Can you work these out from the model? Positions are in its coordinate system, mm. Face numbers are marked on the shaded views. Give positions to 0.01 mm unless a question says otherwise; leave off trailing zeros. Order: outer loops, then holes, each group sorted by start corner. A loop starts at its lowest first (then second) coordinate and runs counter-clockwise, first axis right, second up.
Item 1: I want a section at A-A, the plane x = 21.5. Write out the boundary of the cut face in (y, z).
Item 2: I'm going to push a flat-ended pin straight in: pin 1 Ø1.8 at (x, y) = (30, 6) entering from +Z. Where does the tip first touch, or does it pass through?
Item 3: If I drill on line 1 along X through (y, z) = (29, 1.4); line 2 along Y through (x, z) = (5, 3.65); line 3 along Y through (x, z) = (29, 0.5), over which ranges is the centre line in solid material (lowest first)?
Item 4: I want a section at D-D, the plane y = 5. Write out the boundary of the cut face in (x, z), then the cut area to 3 significant figures.
Item 5: If we mould it in two halves opening along Y, with no side actions, what happens to the marked faces 1, 2 and 3? For each: +Y half, -Y half, draft (parallel to the pull), parting line (faces both ways), or undercut.
Item 6: I want a section at B-B, the plane y = 17. Write out the boundary of the cut face in (x, z).
Item 7: I want a section at C-C, the plane z = 0.45. Write out the boundary of the cut face in (x, y), then the cut area to 3 significant figures.
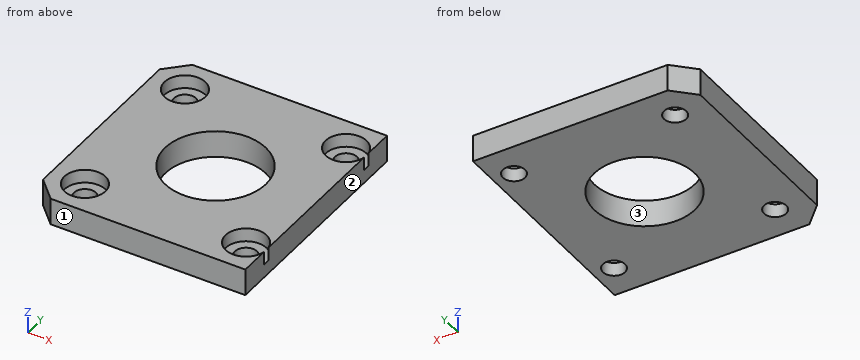
```python
from build123d import *

# Parameters (mm, degrees)
SKETCH_1_R          = 7.5
SKETCH_1_R_2        = 1.65
EXTRUDE_1_DEPTH     = 4
SKETCH_2_R          = 3.05
CUT_EXTRUDE_1_DEPTH = 2


with BuildPart() as part:
    # 草图1 → 凸台-拉伸1 (new body)
    with BuildSketch(Plane.XY):
        Polygon((0, 31), (3, 34), (32, 34), (32, 0), (3, 0), (0, 3), align=None)
        with Locations((17, 17)):
            Circle(SKETCH_1_R, mode=Mode.SUBTRACT)
        with Locations((5, 29)):
            Circle(SKETCH_1_R_2, mode=Mode.SUBTRACT)
        with Locations((29, 29)):
            Circle(SKETCH_1_R_2, mode=Mode.SUBTRACT)
        with Locations((5, 5)):
            Circle(SKETCH_1_R_2, mode=Mode.SUBTRACT)
        with Locations((29, 5)):
            Circle(SKETCH_1_R_2, mode=Mode.SUBTRACT)
    extrude(amount=EXTRUDE_1_DEPTH)

    # 草图2 → 切除-拉伸1 (cut)
    with BuildSketch(Plane.XY.offset(4)):
        with Locations((5, 29)):
            Circle(SKETCH_2_R)
        with Locations((29, 29)):
            Circle(SKETCH_2_R)
        with Locations((5, 5)):
            Circle(SKETCH_2_R)
        with Locations((29, 5)):
            Circle(SKETCH_2_R)
    extrude(amount=-CUT_EXTRUDE_1_DEPTH, mode=Mode.SUBTRACT)


solid = part.part
```
Results list:
1. outline: (0, 0) - (11, 0) - (11, 4) - (0, 4) - close; (23, 0) - (34, 0) - (34, 4) - (23, 4) - close
2. pin 1: stops at z = 2
3. line 1: x = 0 to 3.35, 6.65 to 27.35, 30.65 to 32
3. line 2: y = 0 to 1.95, 8.05 to 25.95, 32.05 to 34
3. line 3: y = 0 to 3.35, 6.65 to 27.35, 30.65 to 34
4. outline: (0, 0) - (3.35, 0) - (3.35, 2) - (1.95, 2) - (1.95, 4) - (0, 4) - close; (6.65, 0) - (27.35, 0) - (27.35, 2) - (25.95, 2) - (25.95, 4) - (8.05, 4) - (8.05, 2) - (6.65, 2) - close; (30.65, 0) - (32, 0) - (32, 2) - (30.65, 2) - close
4. area: 90.5 mm2
5. face 1: -Y half
5. face 2: draft
5. face 3: undercut
6. outline: (0, 0) - (9.5, 0) - (9.5, 4) - (0, 4) - close; (24.5, 0) - (32, 0) - (32, 4) - (24.5, 4) - close
7. outline: (0, 3) - (3, 0) - (32, 0) - (32, 34) - (3, 34) - (0, 31) - close; hole circle Ø3.3 at (5, 5); hole circle Ø3.3 at (5, 29); hole circle Ø15 at (17, 17); hole circle Ø3.3 at (29, 5); hole circle Ø3.3 at (29, 29)
7. area: 868 mm2
